from build123d import *

# Parameters (mm, degrees)
BOSS_EXTRUDE1_DEPTH = 50
SKETCH6_R           = 8.2
CUT_EXTRUDE5_DEPTH  = 75.17
SKETCH7_W           = 50
SKETCH7_H           = 4.818652416
BOSS_EXTRUDE3_DEPTH = 10
SKETCH8_R           = 1.585
CUT_EXTRUDE6_DEPTH  = 10


with BuildPart() as part:
    # Sketch1 → Boss-Extrude1 (new body)
    with BuildSketch(Plane(origin=(0, 0, 0), x_dir=(0, 0, -1), z_dir=(1, 0, 0))):
        Polygon((0, 0), (56.567210857, 0), (56.567210857, 47.465525767), align=None)
    extrude(amount=BOSS_EXTRUDE1_DEPTH)

    # Sketch6 → Cut-Extrude5 (cut)
    with BuildSketch(Plane(origin=(0, 0, -56.567210857), x_dir=(-1, 0, 0), z_dir=(0, 0, -1))):
        with Locations((-38.554443975, 19.83)):
            Circle(SKETCH6_R)
        with Locations((-12.554443975, 19.83)):
            Circle(SKETCH6_R)
    extrude(amount=-CUT_EXTRUDE5_DEPTH, mode=Mode.SUBTRACT)

    # Sketch7 → Boss-Extrude3 (add)
    with BuildSketch(Plane(origin=(0, 0, -56.567210857), x_dir=(-1, 0, 0), z_dir=(0, 0, -1))):
        with Locations((-25, 2.409326208)):
            Rectangle(SKETCH7_W, SKETCH7_H)
    extrude(amount=BOSS_EXTRUDE3_DEPTH)

    # Sketch8 → Cut-Extrude6 (cut)
    with BuildSketch(Plane(origin=(0, 4.818652416, 0), x_dir=(1, 0, 0), z_dir=(0, 1, 0))):
        with Locations(Location((24.681935477, 61.878402744, 0), (0, 0, 270))):
            Circle(SKETCH8_R)
    extrude(amount=-CUT_EXTRUDE6_DEPTH, mode=Mode.SUBTRACT)


solid = part.part
Part model, mm, in its own coordinate system. A direction names the side the tool comes from. Give positions to 0.01 mm unless a question says otherwise; leave off trailing zeros. Write each loop counter-clockwise with the first axis right and the second up, starting at its lowest first coordinate (ties: lowest second). Pieces come first, ordered by that corner, then holes.
1) Cut at D-D on x = 27.5. Write the cut outline in (y, z), then the cut area to 3 significant figures.
Resolved:
outline: (0, -66.57) - (4.82, -66.57) - (4.82, -56.57) - (47.47, -56.57) - (0, 0) - close
area: 1,390 mm2
2) Pin check, flat tips, straight feed: pin 1 (19 mm diameter, centred on x = 38.55, y = 19.83, fed in from -Z); pin 2 (10 mm diameter, centred on x = 40.5, z = -28.5, fed in from -Y); pin 3 (21.5 mm diameter, centred on x = 12.55, y = 19.83, fed in from +Z); pin 4 (3 mm diameter, centred on x = 14, z = -61.5, fed in from +Y). Stop position of each tip, or through.
Resolved:
pin 1: stops at z = -56.57
pin 2: stops at y = 0
pin 3: stops at z = -10.82
pin 4: stops at y = 4.82
3) Two-plate mould, pull along Y, no slides. Class faces 3 (the face through (25, 0, -33)), 4 (the face through (40.332, 11.825, -40.169)), 5 (the face through (0, 18, -40)): released by +Y, released by -Y, zero draft, split by the parting line, or undercut.
Resolved:
face 3: released by -Y
face 4: undercut
face 5: zero draft
4) Cut at B-B on x = 45.5. Write the cut outline in (y, z), then the cut area to 3 significant figures.
Resolved:
outline: (0, -66.57) - (4.82, -66.57) - (4.82, -56.57) - (15.47, -56.57) - (15.47, -18.44) - (0, 0) - close; (24.19, -56.57) - (47.47, -56.57) - (24.19, -28.83) - close
area: 1,100 mm2
5) Cut at A-A on y = 15.5. Write the cut outline in (x, z), then the cut area to 3 significant figures.
Resolved:
outline: (0, -56.57) - (5.59, -56.57) - (5.59, -18.47) - (0, -18.47) - close; (19.52, -56.57) - (31.59, -56.57) - (31.59, -18.47) - (19.52, -18.47) - close; (45.52, -56.57) - (50, -56.57) - (50, -18.47) - (45.52, -18.47) - close
area: 844 mm2
6) Which spindle directions (+Z, -Z, +X, -X, +Y, -Y) get a long thin tool onto all of the face, cutting with end or side? Do faces 1 (the face through (25, 26, -56.567)), 2 (the face through (25.8, 2.4, -63)). Say none if no direction does.
Resolved:
face 1: -Z, +X, -X, +Y
face 2: +Y, -Y
7) Cut at C-C on z = -51. Write the cut outline in (x, y).
Resolved:
outline: (0, 0) - (50, 0) - (50, 42.79) - (0, 42.79) - close; hole circle Ø16.4 at (12.55, 19.83); hole circle Ø16.4 at (38.55, 19.83)
8) Probe L1, parallel to X at y = 19.83, z = -41; L2, parallel to X at y = 24, z = -47; L3, parallel to Y at x = 33, z = -45.5. List the from-to ranges inside material, lowest first.
Resolved:
L1: x = 0 to 4.35, 20.75 to 30.35, 46.75 to 50
L2: x = 0 to 5.49, 19.61 to 31.49, 45.61 to 50
L3: y = 0 to 13.8, 25.86 to 38.18
